The model under review builds one solid part; all positions refer to its coordinate system, in mm. A direction names the side the tool comes from. Give positions to 0.01 mm unless a question says otherwise; leave off trailing zeros. Order: outer loops, then holes, each group sorted by start corner. A loop starts at its lowest first (then second) coordinate and runs counter-clockwise, first axis right, second up. Notation, with made-up numbers: (70.25, -25.5) - (121.25, -25.5) arc R30 cw to (121.25, 1.5) - close; hole circle Ø4 at (15, -0.75). An arc over 180 degrees is marked (long way). Put each result on its own line as item: value.
Autodesk Inventor part; units mm, degrees
ref_plane "Work Plane1" through (0, 25.4, 25.4) normal (0, 1, 0) x (1, 0, 0)
ref_plane "YZ Plane" through (0, 0, 0) normal (1, 0, 0) x (0, 1, 0)
ref_plane "XZ Plane" through (0, 0, 0) normal (0, 1, 0) x (-1, 0, 0)
sketch "Sketch1" plane through (0, 0, 0) normal (0, 1, 0) x (-1, 0, 0)
  circle A0 centre (0, 0) radius 60.325
  dimension "d0" = 120.65
extrude "Extrusion1" add sketch "Sketch1" along normal blind 6.35
sketch "Sketch2" plane through (0, 6.35, 0) normal (0, 1, 0) x (1, 0, 0)
  circle A0 centre (0, 0) radius 60.325
  arc A1 (3.81, 50.8) -> (-3.81, 50.8) centre (0, 50.8) ccw
  arc A2 (-3.81, 25.4) -> (3.81, 25.4) centre (0, 25.4) ccw
  line L0 (-3.81, 50.8) -> (-3.81, 25.4)
  line L1 (3.81, 50.8) -> (3.81, 25.4)
  dimension "d3" = 25.4
  dimension "d4" = 7.62
  dimension "d5" = 50.8
extrude "Extrusion2" cut sketch "Sketch2" against normal blind 5.08 contours L1 A2 L0 A1
sketch "Sketch3" plane through (0, 6.35, 0) normal (0, 1, 0) x (1, 0, 0)
  line L0 (-3.81, 25.4) -> (-3.81, 50.8)
  arc A0 (3.81, 50.8) -> (-3.81, 50.8) centre (0, 50.8) ccw
  line L1 (3.81, 50.8) -> (3.81, 25.4)
  arc A1 (-3.81, 25.4) -> (3.81, 25.4) centre (0, 25.4) ccw
  line L2 (6.35, 25.4) -> (6.35, 50.8)
  arc A2 (6.35, 50.8) -> (-6.35, 50.8) centre (0, 50.8) ccw
  line L3 (-6.35, 50.8) -> (-6.35, 25.4)
  arc A3 (-6.35, 25.4) -> (6.35, 25.4) centre (0, 25.4) ccw
  dimension "d8" = 2.54
extrude "Extrusion3" cut sketch "Sketch3" against normal blind 2.54
sketch "Sketch4" plane through (0, 3.81, 0) normal (0, 1, 0) x (1, 0, 0)
  arc A0 (3.81, 50.8) -> (-3.81, 50.8) centre (0, 50.8) ccw
  line L0 (-2.54, 67.2746) -> (2.54, 67.2746)
  line L1 (2.54, 67.2746) -> (2.54, 48.8018)
  line L2 (2.54, 48.8018) -> (-2.54, 48.8018)
  line L3 (-2.54, 48.8018) -> (-2.54, 67.2746)
  point P0 (0, 0)
  point P1 (0, 48.8018)
  dimension "d11" = 5.08
extrude "Extrusion4" cut sketch "Sketch4" against normal blind 2.54
sketch "Sketch5" plane through (0, 6.35, 0) normal (0, 1, 0) x (1, 0, 0)
  arc A0 (6.35, 50.8) -> (-6.35, 50.8) centre (0, 50.8) ccw
  line L0 (4.445, 43.4525) -> (-4.445, 43.4525)
  line L1 (-4.445, 43.4525) -> (-4.445, 150.3399)
  line L2 (-4.445, 150.3399) -> (4.445, 150.3399)
  line L3 (4.445, 150.3399) -> (4.445, 43.4525)
  point P0 (0, 43.4525)
  dimension "d14" = 8.89
extrude "Extrusion5" cut sketch "Sketch5" against normal blind 2.54
sketch "Sketch6" plane through (0, 1.27, 0) normal (0, 1, 0) x (1, 0, 0)
  arc A0 (-2.54, 53.6398) -> (-3.81, 50.8) centre (0, 50.8) ccw
  arc A1 (-3.81, 25.4) -> (3.81, 25.4) centre (0, 25.4) ccw
  circle A2 centre (0, 50.8) radius 1.524
  circle A3 centre (0, 31.75) radius 1.524
  dimension "d17" = 6.35
  dimension "d18" = 19.05
  dimension "d19" = 3.048
extrude "Extrusion6" cut sketch "Sketch6" against normal through all
sketch "Sketch8" plane through (0, 6.35, 0) normal (0, 1, 0) x (1, 0, 0)
  arc A0 (6.35, 50.8) -> (4.445, 55.3348) centre (0, 50.8) ccw
  circle A1 centre (25.4, 38.1) radius 6.35
  dimension "d25" = 12.7
  dimension "d26" = 25.4
  dimension "d27" = 12.7
extrude "Extrusion8" cut sketch "Sketch8" against normal through all
ref_plane "Work Plane1" through (0, 25.4, 25.4) normal (0, 1, 0) x (1, 0, 0)
sketch "Sketch11" plane through (0, 25.4, 25.4) normal (0, 1, 0) x (1, 0, 0)
  circle A0 centre (0, 0) radius 6.35
  circle A1 centre (0, 0) radius 1.7145
  point P0 (0, 25.4)
  dimension "d41" = 3.429
extrude "Extrusion11" cut sketch "Sketch11" against normal through all contours A1
pattern_circular "Circular Pattern2" count 3 over 360 about axis through (0, 0, 0) along (0, 1, 0) of "Extrusion2", "Extrusion3", "Extrusion4", "Extrusion5", "Extrusion6", "Extrusion8", "Extrusion11"
sketch "Sketch12" plane through (0, 6.35, 0) normal (0, 1, 0) x (1, 0, 0)
  line L0 (6.35, 50.8) -> (6.35, 25.4)
  arc A0 (-6.35, 25.4) -> (6.35, 25.4) centre (0, 25.4) ccw
  line L1 (-6.35, 25.4) -> (-6.35, 50.8)
  line L2 (8.89, 16.51) -> (-8.89, 16.51)
  line L3 (-8.89, 16.51) -> (-8.89, 73.5525)
  line L4 (-8.89, 73.5525) -> (8.89, 73.5525)
  line L5 (8.89, 73.5525) -> (8.89, 16.51)
  dimension "d47" = 2.54
  dimension "d48" = 2.54
  dimension "d49" = 2.54
extrude "Extrusion12" cut sketch "Sketch12" against normal through all keep common part
properties part number "Attachment Point - Female"
(1) The part is to be moulded in two halves that separate along X. For faces 1 (the flat face through (-3.81, 3, -38)), 2 (the flat face through (8.89, 3, -38)), 3 (the flat face through (7, 6.35, -37)), say which applies: pulls with the +X half, pulls with the -X half, needs draft (parallel to the pull), parting line crosses it, or undercut.
The answers:
face 1: undercut
face 2: pulls with the +X half
face 3: needs draft
(2) Clearance check with flat-ended pins moving along their axes: pin 1 Ø3 at (x, y) = (7, 4) entering from -Z; pin 2 Ø4 at (x, z) = (0, -31.75) entering from +Y; pin 3 Ø4 at (x, z) = (3, -46.5) entering from +Y. State where each tip first meets the part, or that it passes through.
The answers:
pin 1: z = -60.07
pin 2: y = 1.27
pin 3: y = 3.81
(3) Take a section at A-A, the plane x = 0. Write out the cut boundary in (y, z) (3 decimals).
The answers:
outline: (0, -60.325) - (1.27, -60.325) - (1.27, -52.324) - (0, -52.324) - close; (0, -49.276) - (1.27, -49.276) - (1.27, -33.274) - (0, -33.274) - close; (0, -30.226) - (1.27, -30.226) - (1.27, -21.59) - (3.81, -21.59) - (3.81, -19.05) - (6.35, -19.05) - (6.35, -16.51) - (0, -16.51) - close
(4) Wall thickness on L1, parallel to Z at x = 0, y = 0.5 (3 decimals); L2, parallel to X at y = 5.5, z = -49.5; L3, parallel to X at y = 0.45, z = -50.8: over which ranges is each line inside the solid? List them lowest first.
The answers:
L1: -60.325 to -52.324, -49.276 to -33.274, -30.226 to -16.51
L2: -8.89 to -6.35, 6.35 to 8.89
L3: -8.89 to -1.52, 1.52 to 8.89
(5) For faces 4 (the flat face through (0, 0, -38)), 5 (the flat face through (6.35, 5, -38)), 6 (the flat face through (4.445, 5, -58)), list the 3-axis set-ups (+Z, -Z, +X, -X, +Y, -Y) from which the entire face can be reached by the end or side of a thin tool; tool diameter is ignored.
The answers:
face 4: +Z, -Z, +X, -X, -Y
face 5: +Y
face 6: -Z, +Y
(6) Take a section at B-B, the plane z = -31.75. Write out the cut boundary in (x, y), then the cut area to 3 significant figures.
The answers:
outline: (-8.89, 0) - (-1.52, 0) - (-1.52, 1.27) - (-3.81, 1.27) - (-3.81, 3.81) - (-6.35, 3.81) - (-6.35, 6.35) - (-8.89, 6.35) - close; (1.52, 0) - (8.89, 0) - (8.89, 6.35) - (6.35, 6.35) - (6.35, 3.81) - (3.81, 3.81) - (3.81, 1.27) - (1.52, 1.27) - close
area: 57.4 mm^2
(7) Take a section at D-D, the plane x = -5. Write out the cut boundary in (y, z), then the cut area to 3 significant figures.
The answers:
outline: (0, -60.12) - (6.35, -60.12) - (6.35, -54.71) - (3.81, -54.71) - (3.81, -21.49) - (6.35, -21.49) - (6.35, -16.51) - (0, -16.51) - close
area: 193 mm^2
